The figure shows three views and two pictorial views of one solid part (mm, origin at its lowest corner). Answer the questions. Round coordinates to 2 decimals unless told otherwise and drop trailing zeros. Write each loop counter-clockwise with the first axis right and the second up, starting at its lowest first coordinate (ties: lowest second). Pieces come first, ordered by that corner, then holes. Notation, with made-up numbers: (58, 16.5) -> (69, 16.5) arc R14 cw to (69, 42.5) -> close; hole circle Ø3 at (40.5, 48.5). An arc over 180 degrees is marked (long way). One line per item, written item: value.
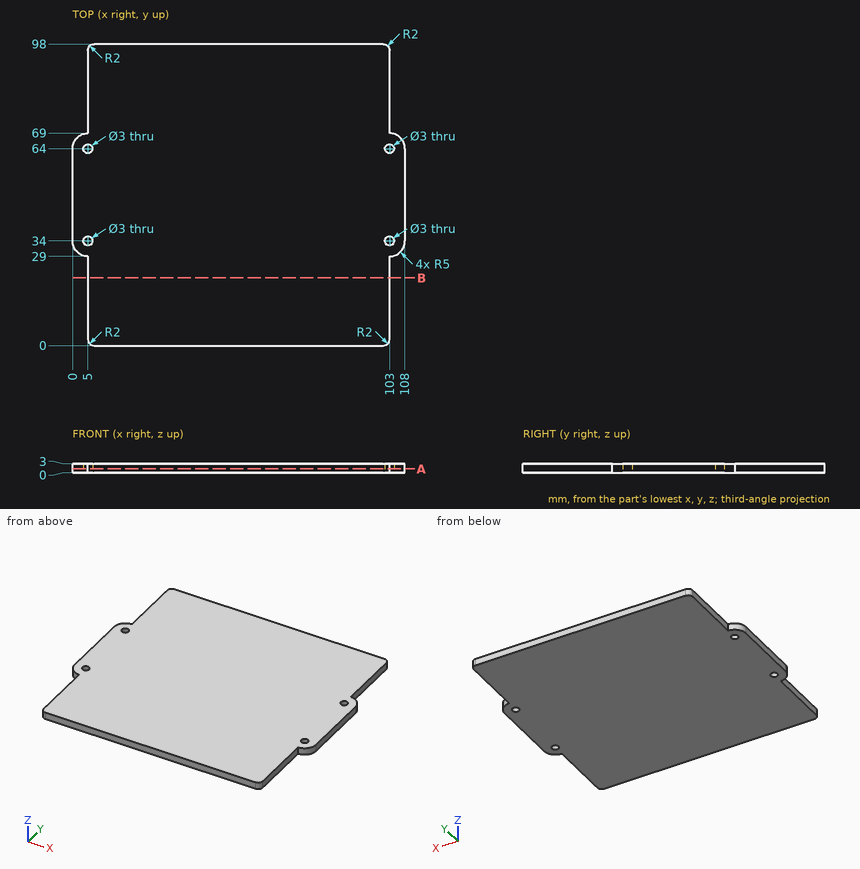
(1) Consider probe 1 along X at (y, z) = (64, 0.7); probe 2 along X at (y, z) = (14.5, 2). Determine where each line is inside the solid, lowest interval first.
Reported:
probe 1: x = 0 to 3.5, 6.5 to 101.5, 104.5 to 108
probe 2: x = 5 to 103
(2) Find section A-A on z = 1.3. Give the number of separate pieces and of enclosed holes in the cut face, plus the area to 3 significant figures.
Reported:
separate pieces: 1
enclosed holes: 4
area: 9,950 mm2
(3) Flat-ended cylindrical pins translate along their axes: pin 1 Ø2.5 at (x, y) = (103, 64) entering from -Z; pin 2 Ø1 at (y, z) = (25, 0.5) entering from -X; pin 3 Ø1.5 at (y, z) = (9.5, 2) entering from +X. Find the tip coordinate at first contact, or state that the pin passes through.
Reported:
pin 1: passes through
pin 2: stops at x = 5
pin 3: stops at x = 103
(4) Find section B-B on y = 22. Give the vertices of the cut face in (x, z), plus the area to 3 significant figures.
Reported:
outline: (5, 0) -> (103, 0) -> (103, 3) -> (5, 3) -> close
area: 294 mm2
